Can you work these out from the model? Positions are in its coordinate system, mm. Face numbers are marked on the shaded views. Give positions to 0.01 mm unless a question says otherwise; leave off trailing zeros. Loops run counter-clockwise (first coordinate to the right, second up) from the corner with the lowest first, then second, coordinate; pieces in that order, holes last. Notation, with made-up numbers: (-19.5, 47) - (35.5, 47) arc R15 ccw to (35.5, 76) - close; hole circle Ø10 at (53, 18). An arc over 180 degrees is marked (long way). Answer in a Markdown table with one row per item.
from build123d import *

# Parameters (mm, degrees)
SKETCH1_R           = 40
SKETCH1_R_2         = 30
SKETCH1_R_3         = 2.5
BOSS_EXTRUDE1_DEPTH = 50
SKETCH2_R           = 43
SKETCH2_R_2         = 30
BOSS_EXTRUDE2_DEPTH = 5
SKETCH3_R           = 43
SKETCH3_R_2         = 30
SKETCH3_R_3         = 2.5
BOSS_EXTRUDE3_DEPTH = 5


with BuildPart() as part:
    # Sketch1 → Boss-Extrude1 (new body)
    with BuildSketch(Plane.XY):
        Circle(SKETCH1_R)
        Circle(SKETCH1_R_2, mode=Mode.SUBTRACT)
        with Locations((0, 35)):
            Circle(SKETCH1_R_3, mode=Mode.SUBTRACT)
        with Locations((18.922428611, 29.443873649)):
            Circle(SKETCH1_R_3, mode=Mode.SUBTRACT)
        with Locations((31.837119837, 14.539525455)):
            Circle(SKETCH1_R_3, mode=Mode.SUBTRACT)
        with Locations((34.643750466, -4.98101934)):
            Circle(SKETCH1_R_3, mode=Mode.SUBTRACT)
        with Locations((26.451235102, -22.920125688)):
            Circle(SKETCH1_R_3, mode=Mode.SUBTRACT)
        with Locations((9.860639489, -33.582254077)):
            Circle(SKETCH1_R_3, mode=Mode.SUBTRACT)
        with Locations((-9.860639489, -33.582254077)):
            Circle(SKETCH1_R_3, mode=Mode.SUBTRACT)
        with Locations((-26.451235102, -22.920125688)):
            Circle(SKETCH1_R_3, mode=Mode.SUBTRACT)
        with Locations((-34.643750466, -4.98101934)):
            Circle(SKETCH1_R_3, mode=Mode.SUBTRACT)
        with Locations((-31.837119837, 14.539525455)):
            Circle(SKETCH1_R_3, mode=Mode.SUBTRACT)
        with Locations((-18.922428611, 29.443873649)):
            Circle(SKETCH1_R_3, mode=Mode.SUBTRACT)
    extrude(amount=BOSS_EXTRUDE1_DEPTH)

    # Sketch2 → Boss-Extrude2 (add)
    with BuildSketch(Plane(origin=(0, 0, 0), x_dir=(-1, 0, 0), z_dir=(0, 0, -1))):
        Circle(SKETCH2_R)
        Circle(SKETCH2_R_2, mode=Mode.SUBTRACT)
    extrude(amount=BOSS_EXTRUDE2_DEPTH)

    # Sketch3 → Boss-Extrude3 (add)
    with BuildSketch(Plane.XY.offset(50)):
        Circle(SKETCH3_R)
        Circle(SKETCH3_R_2, mode=Mode.SUBTRACT)
        with Locations((31.837119837, 14.539525455)):
            Circle(SKETCH3_R_3, mode=Mode.SUBTRACT)
        with Locations((34.643750466, -4.98101934)):
            Circle(SKETCH3_R_3, mode=Mode.SUBTRACT)
        with Locations((26.451235102, -22.920125688)):
            Circle(SKETCH3_R_3, mode=Mode.SUBTRACT)
        with Locations((9.860639489, -33.582254077)):
            Circle(SKETCH3_R_3, mode=Mode.SUBTRACT)
        with Locations((-9.860639489, -33.582254077)):
            Circle(SKETCH3_R_3, mode=Mode.SUBTRACT)
        with Locations((-26.451235102, -22.920125688)):
            Circle(SKETCH3_R_3, mode=Mode.SUBTRACT)
        with Locations((-34.643750466, -4.98101934)):
            Circle(SKETCH3_R_3, mode=Mode.SUBTRACT)
        with Locations((-31.837119837, 14.539525455)):
            Circle(SKETCH3_R_3, mode=Mode.SUBTRACT)
        with Locations((-18.922428611, 29.443873649)):
            Circle(SKETCH3_R_3, mode=Mode.SUBTRACT)
        with Locations((0, 35)):
            Circle(SKETCH3_R_3, mode=Mode.SUBTRACT)
        with Locations((18.922428611, 29.443873649)):
            Circle(SKETCH3_R_3, mode=Mode.SUBTRACT)
    extrude(amount=BOSS_EXTRUDE3_DEPTH)


solid = part.part
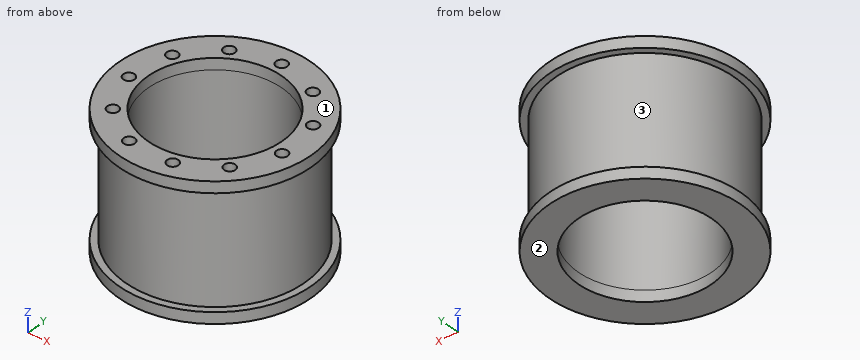
Q1. If we mould it in two halves opening along Z, with no side actions, what happens to the marked faces 1, 2 and 3? For each: released by +Z, released by -Z, zero draft, split by the parting line, or undercut.
Checked values:
| item | result |
|---|---|
| face 1 | released by +Z |
| face 2 | released by -Z |
| face 3 | undercut |
Q2. For pin 1 (10 mm diameter, centred on x = -2, z = 14, fed in from -Y); pin 2 (1.5 mm diameter, centred on x = -27.5, y = -23, fed in from +Z); pin 3 (1.5 mm diameter, centred on x = -22, z = 24, fed in from +Y), each with a flat end and sliding along its axis, tell me the tip position at first contact or that it passes through.
Checked values:
| item | result |
|---|---|
| pin 1 | stops at y = -40 |
| pin 2 | stops at z = 0 |
| pin 3 | stops at y = 33.89 |
Q3. If I drill on line 1 (Y direction, x = 21, z = 40); line 2 (X direction, y = -25, z = 11.5); line 3 (Y direction, x = -1, z = 41.5), over which ranges is the centre line in solid material (lowest first)? Write a range as [from, to].
Checked values:
| item | result |
|---|---|
| line 1 | y = [-34.04, -21.42], [21.42, 28.05], [30.83, 34.04] |
| line 2 | x = [-31.22, -27.84], [-25.06, -16.58], [16.58, 25.06], [27.84, 31.22] |
| line 3 | y = [-39.99, -29.98], [29.98, 32.71], [37.29, 39.99] |
Q4. Imagine slicing it at A-A, the plane x = 0. Write out the boundary of the cut face in (y, z), and give its area (3 significant figures).
Checked values:
| item | result |
|---|---|
| outline | (-43, -5) - (-30, -5) - (-30, 55) - (-43, 55) - (-43, 50) - (-40, 50) - (-40, 0) - (-43, 0) - close; (30, -5) - (43, -5) - (43, 0) - (40, 0) - (40, 50) - (43, 50) - (43, 55) - (37.5, 55) - (37.5, 0) - (32.5, 0) - (32.5, 55) - (30, 55) - close |
| area | 985 mm² |
Q5. Imagine slicing it at B-B, the plane y = 0. Write out the boundary of the cut face in (x, z), and give its area (3 significant figures).
Checked values:
| item | result |
|---|---|
| outline | (-43, -5) - (-30, -5) - (-30, 55) - (-43, 55) - (-43, 50) - (-40, 50) - (-40, 0) - (-43, 0) - close; (30, -5) - (43, -5) - (43, 0) - (40, 0) - (40, 50) - (43, 50) - (43, 55) - (30, 55) - close |
| area | 1,260 mm² |
Q6. Imagine slicing it at C-C, the plane z = 1.5. Count the separate pieces of the cut face and the enclosed holes in it, and give its area (3 significant figures).
Checked values:
| item | result |
|---|---|
| separate pieces | 1 |
| enclosed holes | 12 |
| area | 1,980 mm² |
Q7. Imagine slicing it at D-D, the plane y = 35. Write out the boundary of the cut face in (x, z), and give its area (3 significant figures).
Checked values:
| item | result |
|---|---|
| outline | (-24.98, -5) - (24.98, -5) - (24.98, 0) - (19.36, 0) - (19.36, 50) - (24.98, 50) - (24.98, 55) - (2.5, 55) - (2.5, 0) - (-2.5, 0) - (-2.5, 55) - (-24.98, 55) - (-24.98, 50) - (-19.36, 50) - (-19.36, 0) - (-24.98, 0) - close |
| area | 2,160 mm² |
